Could you check a few things on this drawing? It's one solid part, dimensions in mm from its lowest x, y, z. A direction names the side the tool comes from. Coordinates: 2 decimals unless noted, no trailing zeros. Loops run counter-clockwise (first coordinate to the right, second up) from the corner with the lowest first, then second, coordinate; pieces in that order, holes last. Notation, with made-up numbers: M -2,59.5 L 3,59.5 A19 cw 3,91.5 Z; hole C -21.75,78.5 d6. An arc over 180 degrees is marked long. Answer as a JSON object with one key per item and string values. Group by question number.
Item 1: I'm going to push flat-ended pins straight in: pin 1 Ø4 at (x, z) = (195, 20) entering from +Y; pin 2 Ø8 at (y, z) = (21, 15) entering from +X; pin 3 Ø10 at (x, z) = (15, 20) entering from -Y; pin 4 Ø9 at (x, z) = (164.2, 20) entering from +Y. Where does each tip first touch, or does it pass through?
Item 2: Suppose I cut it at A-A (x = 195). Write out the boundary of the cut face in (y, z) (3 decimals).
Item 3: Suppose I cut it at D-D (x = 164.2). Write out the boundary of the cut face in (y, z).
Item 4: If I drill on line 1 (Z direction, x = 45.8, y = 3.5); line 2 (Y direction, x = 185, z = 29); line 3 (Y direction, x = 56.5, z = 16), over which ranges is the centre line in solid material (lowest first)?
Item 5: Suppose I cut it at B-B (z = 20). Write out the boundary of the cut face in (x, y) (3 decimals), then the cut area to 3 significant figures.
Item 6: Which directions (+Z, -Z, +X, -X, +Y, -Y) give clear straight access to the entire face, cutting with the end or side of a thin tool? Please do the marked faces 1, 2 and 3.
Item 7: Suppose I cut it at C-C (z = 29). Write out the boundary of the cut face in (x, y), then the cut area to 3 significant figures.
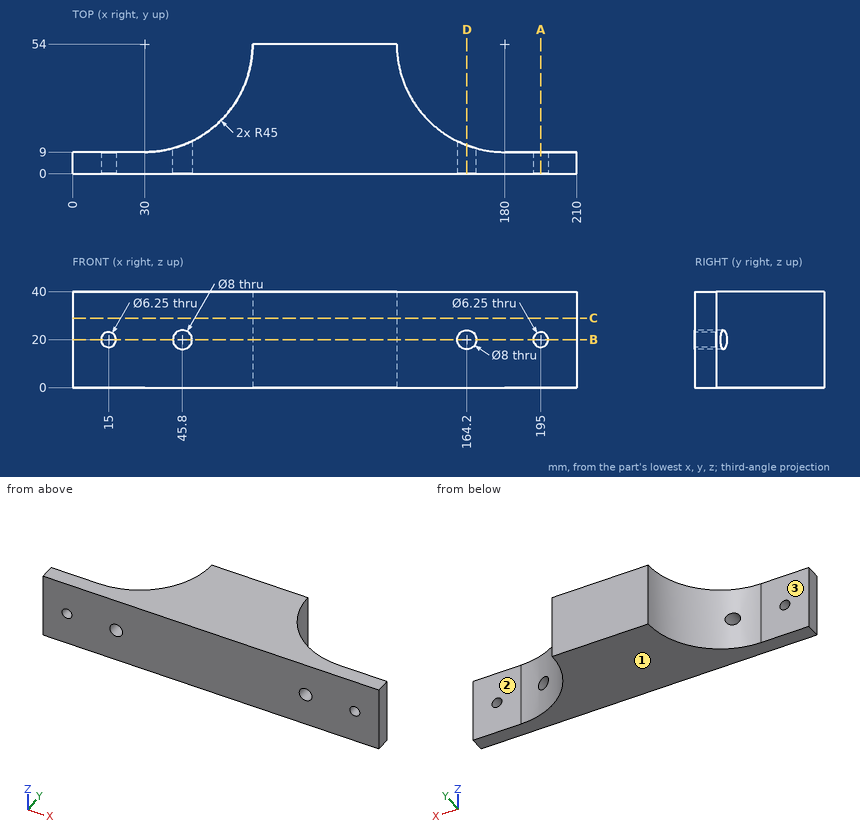
From the geometry:
{
 "1": {"pin 1": "through", "pin 2": "x = 154.39", "pin 3": "y = 0", "pin 4": "y = 13.84"},
 "2": {"outline": "M 0,0 L 9,0 L 9,16.875 L 0,16.875 Z; M 0,23.125 L 9,23.125 L 9,40 L 0,40 Z"},
 "3": {"outline": "M 0,0 L 11.86,0 L 11.86,16 L 0,16 Z; M 0,24 L 11.86,24 L 11.86,40 L 0,40 Z"},
 "4": {"line 1": "0 to 16, 24 to 40", "line 2": "0 to 9", "line 3": "0 to 17.63"},
 "5": {"outline": "M 0,0 L 11.875,0 L 11.875,9 L 0,9 Z; M 18.125,0 L 41.8,0 L 41.8,10.575 A45 cw 30,9 L 18.125,9 Z; M 49.8,0 L 160.2,0 L 160.2,13.59 A45 cw 135,54 L 75,54 A45 cw 49.8,13.59 Z; M 168.2,0 L 191.875,0 L 191.875,9 L 180,9 A45 cw 168.2,10.575 Z; M 198.125,0 L 210,0 L 210,9 L 198.125,9 Z", "area": "5,160 mm2"},
 "6": {"face 1": "-Z, +X, -X, +Y, -Y", "face 2": "+Z, -Z, +X, +Y", "face 3": "+Z, -Z, -X, +Y"},
 "7": {"outline": "M 0,0 L 210,0 L 210,9 L 180,9 A45 cw 135,54 L 75,54 A45 cw 30,9 L 0,9 Z", "area": "5,460 mm2"}
}
